The listing builds one solid part. Answer for the finished solid, in the listing's coordinates (mm). Give positions to 0.01 mm unless a question says otherwise; leave off trailing zeros. Order: outer loops, then holes, each group sorted by start corner. A loop starts at its lowest first (then second) coordinate and runs counter-clockwise, first axis right, second up. Notation, with made-up numbers: (75.5, 36.5) - (104.5, 36.5) arc R19 cw to (104.5, 42.5) - close; hole circle Ø9 at (-32, -5.5). An arc over 180 degrees is marked (long way). Answer in a Markdown table with one row per item.
Autodesk Inventor part; units mm, degrees
ref_plane "YZ Plane" through (0, 0, 0) normal (1, 0, 0) x (0, 1, 0)
ref_plane "XZ Plane" through (0, 0, 0) normal (0, 1, 0) x (-1, 0, 0)
ref_plane "XY Plane" through (0, 0, 0) normal (0, 0, 1) x (1, 0, 0)
sketch "スケッチ1" plane through (0, 0, 0) normal (0, 1, 0) x (-1, 0, 0)
  circle A0 centre (0, 0) radius 56.5
  circle A1 centre (0, 0) radius 44.5
  dimension "d0" = 113
  dimension "d1" = 89
extrude "押し出し1" add sketch "スケッチ1" along normal blind 1
sketch "スケッチ2" plane through (0, 1, 0) normal (0, 1, 0) x (1, 0, 0)
  circle A0 centre (0, 0) radius 50.75
  point P0 (-50.75, 0)
  point P1 (0, -50.75)
  point P2 (50.75, 0)
  point P3 (0, 50.75)
  dimension "d4" = 101.5
  dimension "d7" = 360
hole "穴1" at (-50.75, 1, 0) at (0, 1, 50.75) at (50.75, 1, 0) at (0, 1, -50.75) direction (0, -1, 0) diameter 4.3 end through all
properties part number "basespacer1"
Item 1: Find section D-D on z = -33. Write down the section's boundary in (x, y), then the cut area to 3 significant figures.
Answer block:
| item | result |
|---|---|
| outline | (-45.86, 0) - (-29.85, 0) - (-29.85, 1) - (-45.86, 1) - close; (29.85, 0) - (45.86, 0) - (45.86, 1) - (29.85, 1) - close |
| area | 32.0 mm² |
Item 2: Find section C-C on y = 0.3. Write down the section's boundary in (x, z), then the cut area to 3 significant figures.
Answer block:
| item | result |
|---|---|
| outline | circle Ø113 at (0, 0); hole circle Ø4.3 at (-50.75, 0); hole circle Ø89 at (0, 0); hole circle Ø4.3 at (0, -50.75); hole circle Ø4.3 at (0, 50.75); hole circle Ø4.3 at (50.75, 0) |
| area | 3,750 mm² |
Item 3: Consider line 1 (Z direction, x = -50.75, y = 0.45); line 2 (Z direction, x = 38.5, y = 0.75); line 3 (X direction, y = 0.5, z = 30). Determine where each line is inside the solid, lowest interval first.
Answer block:
| item | result |
|---|---|
| line 1 | -24.83 to -2.15, 2.15 to 24.83 |
| line 2 | -41.35 to -22.32, 22.32 to 41.35 |
| line 3 | -47.88 to -32.87, 32.87 to 47.88 |
Item 4: This flat-tipped pin is pushed along its axis until it touches: P1, Ø3.5, axis at x = 0, z = 50.75, coming from the +Y side. Where does it stop, or does it pass through?
Answer block:
| item | result |
|---|---|
| P1 | through |
Item 5: Find section B-B on x = 42. Write down the section's boundary in (y, z).
Answer block:
| item | result |
|---|---|
| outline | (0, -37.79) - (1, -37.79) - (1, -14.71) - (0, -14.71) - close; (0, 14.71) - (1, 14.71) - (1, 37.79) - (0, 37.79) - close |
Item 6: Determine the mould class of faces 1 (the face through (-52.56, 0.49, 1.16)), 2 (the face through (34, 1, 30)), 3 (the face through (-30.374, 0.493, -47.641)) for opening direction X: pulls with the +X half, pulls with the -X half, needs draft (parallel to the pull), parting line crosses it, or undercut.
Answer block:
| item | result |
|---|---|
| face 1 | undercut |
| face 2 | needs draft |
| face 3 | parting line crosses it |
Item 7: Find section A-A on z = 0. Write down the section's boundary in (x, y), then the cut area to 3 significant figures.
Answer block:
| item | result |
|---|---|
| outline | (-56.5, 0) - (-52.9, 0) - (-52.9, 1) - (-56.5, 1) - close; (-48.6, 0) - (-44.5, 0) - (-44.5, 1) - (-48.6, 1) - close; (44.5, 0) - (48.6, 0) - (48.6, 1) - (44.5, 1) - close; (52.9, 0) - (56.5, 0) - (56.5, 1) - (52.9, 1) - close |
| area | 15.4 mm² |
